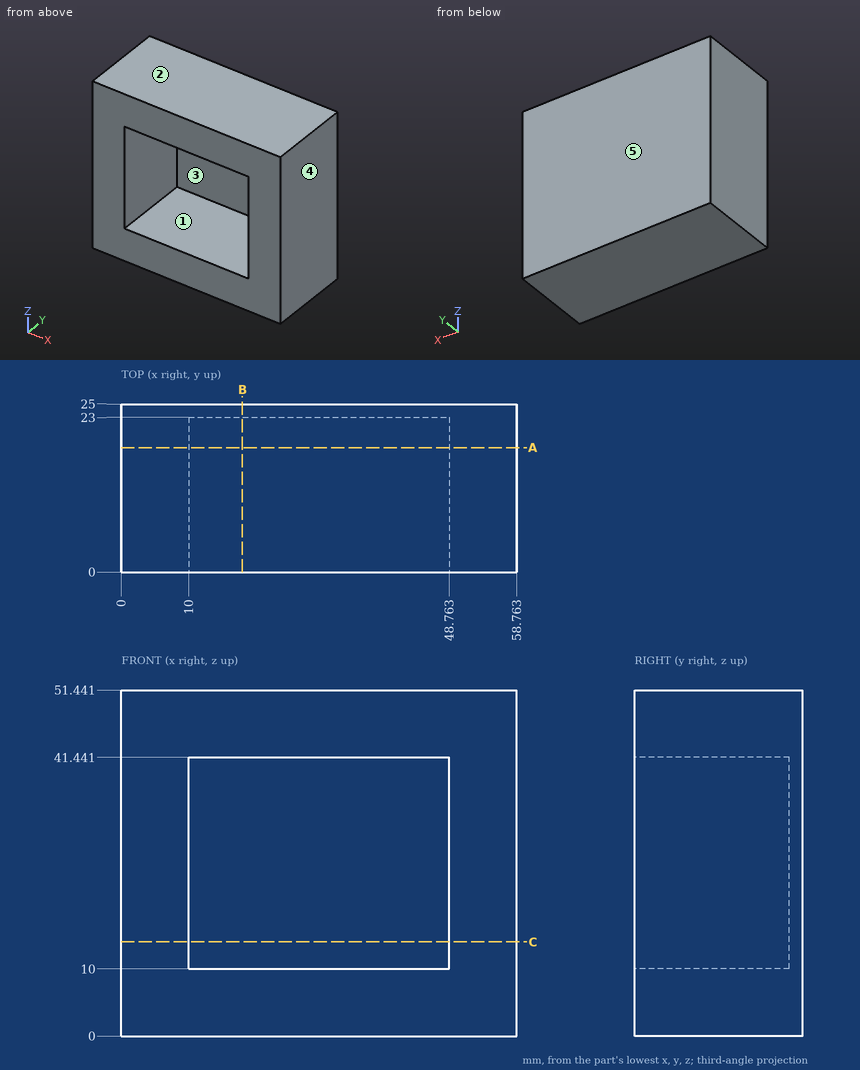
Answer from the drawing. Dimensions are ordinates in mm from the lowest x, y and z of the part. A direction names the side the tool comes from. Give positions to 0.01 mm unless a question says otherwise; leave off trailing zeros. Order: outer loops, then holes, each group sorted by start corner. A loop starts at its lowest first (then second) coordinate and runs counter-clockwise, first axis right, second up.
(1) Straight lines are drawn through the part: L1, parallel to X at y = 12, z = 37; L2, parallel to Z at x = 39, y = 3; L3, parallel to Y at x = 15.5, z = 30. For each, find the intervals that lie inside material, in ascending order.
(2) Given pin 1 (15.5 mm diameter, centred on x = 30, z = 23, fed in from -Y); pin 2 (5 mm diameter, centred on x = 48.5, y = 12, fed in from -Z), each flat-ended and moving along its own axis, determine where each tip first touches the part or whether it passes through.
(3) For the marked faces 1 and 2, determine the directions among +Z, -Z, +X, -X, +Y, -Y from which every point of the face is accessible in a straight line to the end or side of a thin tool.
(4) Find section C-C (z = 14). Give the vertices of the cut face in (x, y).
(5) For a pull along X with two mould halves and no side action, classify the marked faces 3, 4 and 5 as released by +X, released by -X, zero draft, split by the parting line, or undercut.
(6) Find section A-A (y = 18.5). Give the vertices of the cut face in (x, z), plus the area to 3 significant figures.
(7) Find section B-B (x = 18). Give the vertices of the cut face in (y, z), plus the area to 3 significant figures.
Result sheet:
1. L1: x = 0 to 10, 48.76 to 58.76
1. L2: z = 0 to 10, 41.44 to 51.44
1. L3: y = 23 to 25
2. pin 1: stops at y = 23
2. pin 2: stops at z = 0
3. face 1: -Y
3. face 2: +Z, +X, -X, +Y, -Y
4. outline: (0, 0) - (10, 0) - (10, 23) - (48.76, 23) - (48.76, 0) - (58.76, 0) - (58.76, 25) - (0, 25) - close
5. face 3: undercut
5. face 4: released by +X
5. face 5: zero draft
6. outline: (0, 0) - (58.76, 0) - (58.76, 51.44) - (0, 51.44) - close; hole (10, 10) - (48.76, 10) - (48.76, 41.44) - (10, 41.44) - close
6. area: 1,800 mm2
7. outline: (0, 0) - (25, 0) - (25, 51.44) - (0, 51.44) - (0, 41.44) - (23, 41.44) - (23, 10) - (0, 10) - close
7. area: 563 mm2
